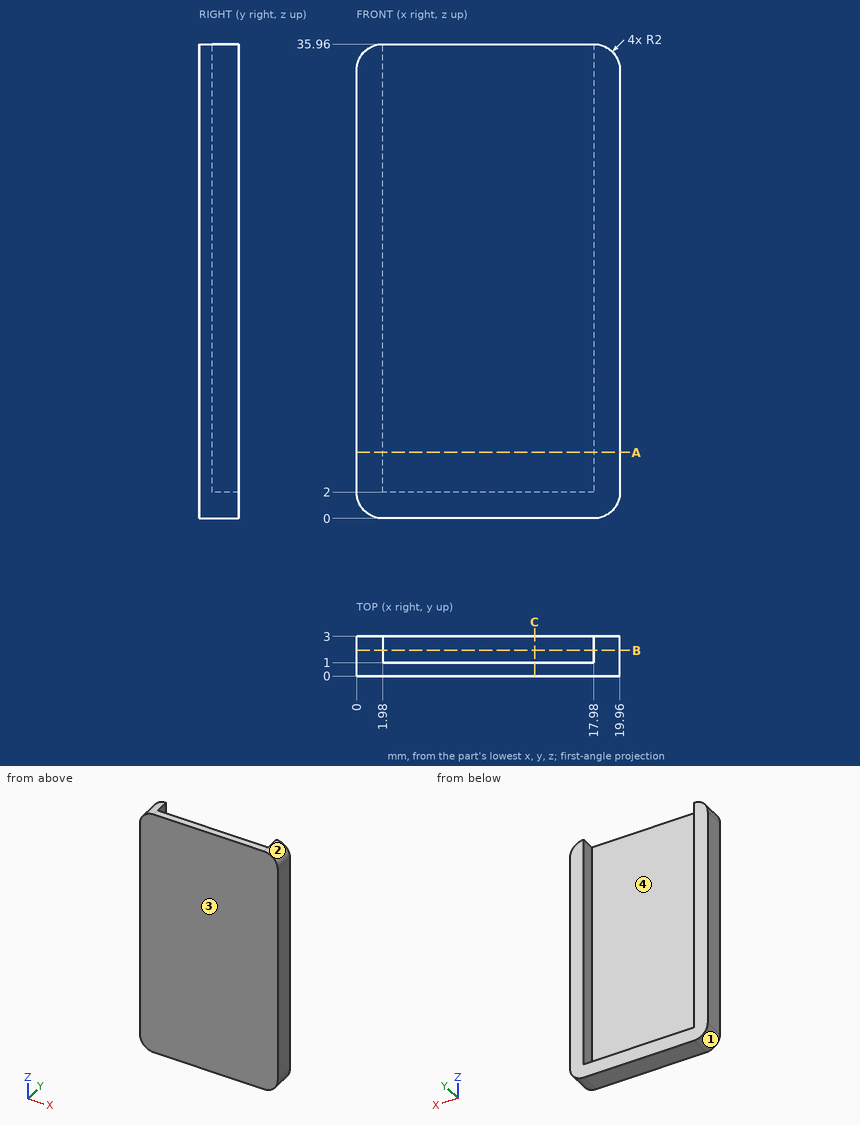
Geometry: see drawing. Coordinates: mm, zero at the bounding-box minimum. Give positions to 0.01 mm unless a question says otherwise; leave off trailing zeros. Loops run counter-clockwise (first coordinate to the right, second up) from the corner with the lowest first, then second, coordinate; pieces in that order, holes last. Notation, with made-up numbers: (14.5, -19.5) - (70.5, -19.5) arc R29 cw to (70.5, 14.5) - close; hole circle Ø7 at (-38.75, 11). An arc over 180 degrees is marked (long way). Use CSV: the item, a comma, the result in double quotes. Start each with the question number.
Item 1: Section A-A on z = 5. Return loops of the section in (x, y).
Item 2: Section B-B on y = 1.95. Return loops of the section in (x, z).
Item 3: Line query: line 1 (X direction, y = 2.5, z = 11); line 2 (Z direction, x = 5.75, y = 2.8); line 3 (Y direction, x = 13, z = 32). Output: solid intervals per line, ascending.
Item 4: Section C-C on x = 13.5. Return loops of the section in (y, z), then the cut area to 3 significant figures.
Item 5: Mould query, pull axis X, two halves, no side actions, for the marked faces 1, 2, 3 and 4. Classes: pulls with the +X half, pulls with the -X half, needs draft (parallel to the pull), parting line crosses it, or undercut.
Item 6: Contact query for flat-ended pins moving along their axis: P1, Ø6, axis at x = 15.5, z = 13, coming from the +Y side; P2, Ø6, axis at x = 6.5, z = 10, coming from the +Y side. Output: stop coordinate, or through.
Ans:
1,outline,"(0, 0) - (19.96, 0) - (19.96, 3) - (17.98, 3) - (17.98, 1) - (1.98, 1) - (1.98, 3) - (0, 3) - close"
2,outline,"(0, 2) arc R2 ccw to (2, 0) - (17.96, 0) arc R2 ccw to (19.96, 2) - (19.96, 33.96) arc R2 ccw to (17.98, 35.96) - (17.98, 2) - (1.98, 2) - (1.98, 35.96) arc R2 ccw to (0, 33.96) - close"
3,line 1,"x = 0 to 1.98, 17.98 to 19.96"
3,line 2,"z = 0 to 2"
3,line 3,"y = 0 to 1"
4,outline,"(0, 0) - (3, 0) - (3, 2) - (1, 2) - (1, 35.96) - (0, 35.96) - close"
4,area,"40.0 mm2"
5,face 1,"pulls with the -X half"
5,face 2,"pulls with the +X half"
5,face 3,"needs draft"
5,face 4,"undercut"
6,P1,"stops at y = 3"
6,P2,"stops at y = 1"
